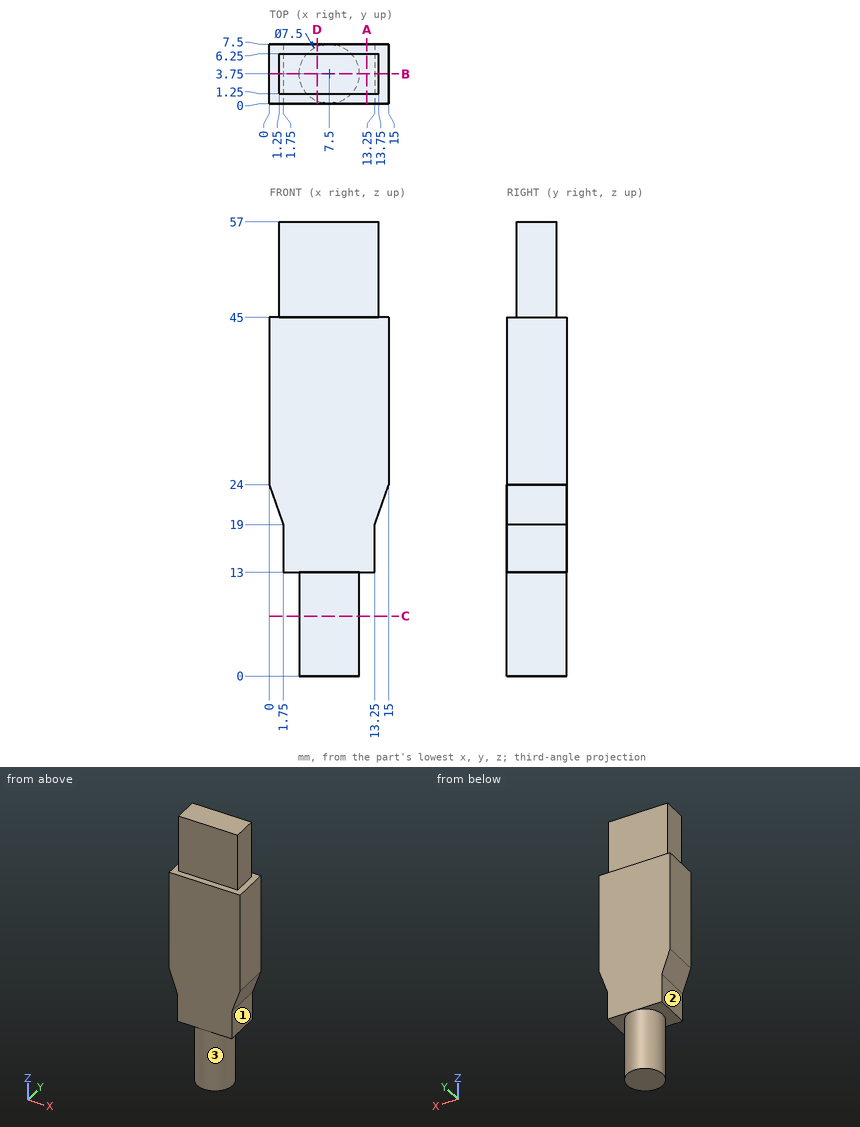
Geometry check sheet. Reference: drawing and pictorial views, mm from the part's lowest x, y, z. A direction names the side the tool comes from. Coordinates: 2 decimals unless noted, no trailing zeros. Order: outer loops, then holes, each group sorted by start corner. A loop starts at its lowest first (then second) coordinate and runs counter-clockwise, first axis right, second up.
Item 1: Section check D-D (x = 6). Enter the section's corners in (y, z), plus the area to 3 significant figures.
Item 2: Tool access check on the marked faces 1, 2 and 3. Record the directions out of +Z, -Z, +X, -X, +Y, -Y that give a thin tool (end or side, any length) a straight path to the whole face; none if there is none.
Item 3: Scan lines: line 1 along Z through (x, y) = (5, 7); line 2 along X through (y, z) = (4, 3); line 3 along X through (y, z) = (6, 19). Record each from-to range of solid material in increasing order.
Item 4: Section check C-C (z = 7.5). Enter the section's corners in (x, y).
Item 5: Section check A-A (x = 12.25). Enter the section's corners in (y, z), plus the area to 3 significant figures.
Item 6: Section check B-B (y = 3.75). Enter the section's corners in (x, z), plus the area to 3 significant figures.
Item 7: Depth check by flat-ended pin: pin 1 (3.5 mm diameter, centred on x = 9.5, z = 53, fed in from +Y); pin 2 (2 mm diameter, centred on y = 3, z = 37.5, fed in from -X); pin 3 (2.5 mm diameter, centred on y = 2.5, z = 50.5, fed in from -X); pin 4 (1.8 mm diameter, centred on y = 5, z = 17.5, fed in from -X). Enter the tip coordinate at first touch or a pass-through.
Check sheet entries:
1. outline: (0, 13) - (0.31, 13) - (0.31, 0) - (7.19, 0) - (7.19, 13) - (7.5, 13) - (7.5, 45) - (6.25, 45) - (6.25, 57) - (1.25, 57) - (1.25, 45) - (0, 45) - close
1. area: 389 mm2
2. face 1: -Z, +X, +Y, -Y
2. face 2: -Z, -X, +Y, -Y
2. face 3: -Z
3. line 1: z = 13 to 45
3. line 2: x = 3.76 to 11.24
3. line 3: x = 1.75 to 13.25
4. outline: circle Ø7.5 at (7.5, 3.75)
5. outline: (0, 13) - (7.5, 13) - (7.5, 45) - (6.25, 45) - (6.25, 57) - (1.25, 57) - (1.25, 45) - (0, 45) - close
5. area: 300 mm2
6. outline: (0, 24) - (1.75, 19) - (1.75, 13) - (3.75, 13) - (3.75, 0) - (11.25, 0) - (11.25, 13) - (13.25, 13) - (13.25, 19) - (15, 24) - (15, 45) - (13.75, 45) - (13.75, 57) - (1.25, 57) - (1.25, 45) - (0, 45) - close
6. area: 698 mm2
7. pin 1: stops at y = 6.25
7. pin 2: stops at x = 0
7. pin 3: stops at x = 1.25
7. pin 4: stops at x = 1.75
